```python
from build123d import *

# Parameters (mm, degrees)
BOSS_EXTRUDE1_DEPTH = 12.7
FILLET2_R           = 0.635
FILLET3_R           = 1.27
FILLET4_R           = 0.508


with BuildPart() as part:
    # Sketch1 → Boss-Extrude1 (new body)
    with BuildSketch(Plane(origin=(0, 0, 0), x_dir=(1, 0, 0), z_dir=(0, 1, 0))):
        with BuildLine():
            Line((17.075, 0), (17.075, -14.88542834))
            Line((17.075, -14.88542834), (20.885, -14.88542834))
            Line((20.885, -14.88542834), (20.885, 10.51457166))
            Line((20.885, 10.51457166), (20.885, 11.27657166))
            Line((20.885, 11.27657166), (18.345, 11.27657166))
            Line((18.345, 11.27657166), (20.885, 13.81657166))
            Line((20.885, 13.81657166), (22.085, 13.81657166))
            Line((22.085, 13.81657166), (22.085, 10.51457166))
            Line((22.085, 10.51457166), (22.085, -16.08542834))
            Line((22.085, -16.08542834), (15.875, -16.08542834))
            Line((15.875, -16.08542834), (15.875, 0))
            ThreePointArc((15.875, 0), (-15.811372489, 1.419903166), (15.621, -2.828424296))
            Line((15.621, -2.828424296), (15.621, -6.89492451))
            ThreePointArc((15.621, -6.89492451), (-16.707546199, 3.52328327), (17.075, 0))
        make_face()
    extrude(amount=BOSS_EXTRUDE1_DEPTH)

    # Fillet2
    fillet2_edges = [part.edges().sort_by_distance(p)[0] for p in [
        (17.075, 6.35, 14.88542834),
        (20.885, 6.35, 14.88542834),
    ]]
    fillet(fillet2_edges, radius=FILLET2_R)

    # Fillet3
    fillet3_edges = [part.edges().sort_by_distance(p)[0] for p in [
        (22.085, 6.35, 16.08542834),
        (15.875, 6.35, 16.08542834),
    ]]
    fillet(fillet3_edges, radius=FILLET3_R)

    # Fillet4
    fillet4_edges = [part.edges().sort_by_distance(p)[0] for p in [
        (15.621, 6.35, 2.828424296),
    ]]
    fillet(fillet4_edges, radius=FILLET4_R)


solid = part.part
```
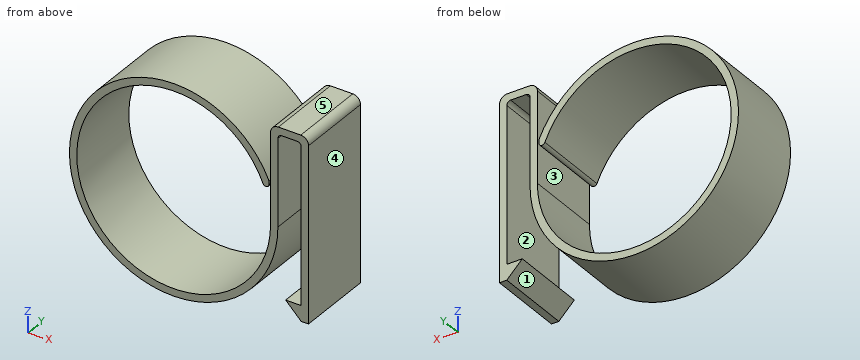
Source: CAD feature listing. Evaluate the final solid. Frame: model axes, mm. Face numbers are marked on the shaded views. A direction names the side the tool comes from. Give positions to 0.01 mm unless a question says otherwise; leave off trailing zeros. Write each loop counter-clockwise with the first axis right and the second up, starting at its lowest first coordinate (ties: lowest second). Pieces come first, ordered by that corner, then holes.
1. Section query A-A (x = 0). Return the cut outline in (y, z) (3 decimals).
2. Access query for the marked faces 1 and 2. Directions: +Z, -Z, +X, -X, +Y, -Y. A direction counts if a zero-diameter tool reaches every point of the face in a straight line with its end or side. Return the directions, or none.
3. Material intervals for line 1 along X through (y, z) = (8, 0) (3 decimals); line 2 along X through (y, z) = (7.75, -4) (3 decimals); line 3 along Z through (x, y) = (0, 8) (3 decimals), sorted ascending.
4. Section query C-C (y = 5.5). Return the cut outline in (x, z) (3 decimals), then the cut area to 3 significant figures.
5. First-contact query: pin 1 (6.5 mm diameter, centred on y = 9, z = 7.5, fed in from -X); pin 2 (1.1 mm diameter, centred on x = 18.5, y = 7, fed in from +Z); pin 3 (1 mm diameter, centred on x = 21.5, y = 7.5, fed in from -Z). Flat tips, straight axial feed; report the tip coordinate or a pass-through.
6. Section query D-D (z = 4.5). Return the cut outline in (x, y) (3 decimals), then the cut area to 3 significant figures.
7. Pull-direction query (X, two-part tool) for the marked faces 3, 4 and 5; classes: +X half, -X half, draft (parallel to the pull), parting line (faces both ways), or undercut.
8. Section query B-B (z = -5). Return the cut outline in (x, y) (3 decimals).
Output values:
1. outline: (0, -17.075) - (12.7, -17.075) - (12.7, -15.875) - (0, -15.875) - close; (0, 15.875) - (12.7, 15.875) - (12.7, 17.075) - (0, 17.075) - close
2. face 1: -Z, +Y, -Y
2. face 2: +Y, -Y
3. line 1: x = -17.075 to -15.875, 15.875 to 17.075, 20.885 to 22.085
3. line 2: x = -16.6 to -15.363, 15.363 to 16.6, 20.885 to 22.085
3. line 3: z = -17.075 to -15.875, 15.875 to 17.075
4. outline: (14.644, 6.128) arc R0.508 ccw to (15.621, 6.325) - (15.621, 6.895) arc R17.075 ccw (long way) to (17.075, 0) - (17.075, 14.25) arc R0.635 cw to (17.71, 14.885) - (20.25, 14.885) arc R0.635 cw to (20.885, 14.25) - (20.885, -11.277) - (18.345, -11.277) - (20.885, -13.817) - (22.085, -13.817) - (22.085, 14.815) arc R1.27 ccw to (20.815, 16.085) - (17.145, 16.085) arc R1.27 ccw to (15.875, 14.815) - (15.875, 0) arc R15.875 cw (long way) to start
4. area: 179 mm2
5. pin 1: stops at x = -16.54
5. pin 2: stops at z = 16.09
5. pin 3: stops at z = -13.82
6. outline: (-16.471, 0) - (-15.224, 0) - (-15.224, 12.7) - (-16.471, 12.7) - close; (15.875, 0) - (17.075, 0) - (17.075, 12.7) - (15.875, 12.7) - close; (20.885, 0) - (22.085, 0) - (22.085, 12.7) - (20.885, 12.7) - close
6. area: 46.3 mm2
7. face 3: undercut
7. face 4: +X half
7. face 5: draft
8. outline: (-16.327, 0) - (-15.067, 0) - (-15.067, 12.7) - (-16.327, 12.7) - close; (15.067, 0) - (16.327, 0) - (16.327, 12.7) - (15.067, 12.7) - close; (20.885, 0) - (22.085, 0) - (22.085, 12.7) - (20.885, 12.7) - close
